CAD build for the part. Positions are in the model's coordinates, mm. Face numbers are marked on the shaded views. Give positions to 0.01 mm unless a question says otherwise; leave off trailing zeros. Loops run counter-clockwise (first coordinate to the right, second up) from the corner with the lowest first, then second, coordinate; pieces in that order, holes last. Notation, with made-up numbers: M 44,-3.5 L 95,-3.5 A11 cw 95,5.5 Z; hole C 56.25,80 d10. An arc over 180 degrees is marked long. One line per question, with ' | ' between items.
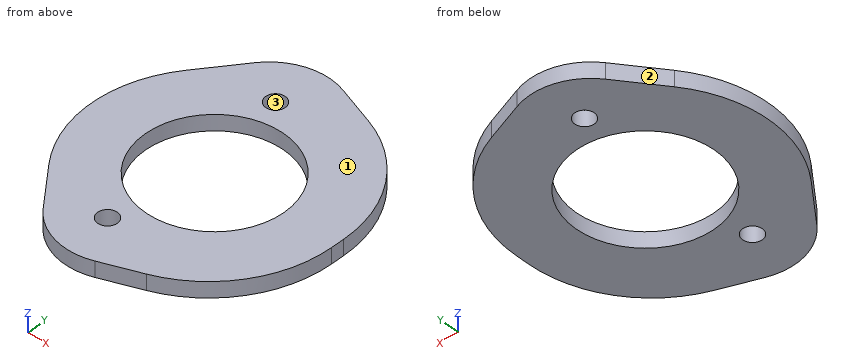
Autodesk Inventor part; units mm, degrees
ref_plane "Work Plane2" through (21.5824, 22.0396, 3.2283) normal (0, 0, 1) x (0.9852, -0.1712, 0)
ref_plane "YZ Plane" through (0, 0, 0) normal (1, 0, 0) x (0, 1, 0)
ref_plane "XZ Plane" through (0, 0, 0) normal (0, 1, 0) x (-1, 0, 0)
ref_plane "Work Plane1" through (0, 0, 0) normal (0, 0, 1) x (1, 0, 0)
sketch "Sketch1" plane through (0, 0, 0) normal (0, 0, 1) x (1, 0, 0)
  line L0 (38.5336, 66.2269) -> (46.4641, 63.2899)
  line L1 (63.0428, 39.4709) -> (63.0428, 36.7291)
  line L2 (46.4641, 12.9101) -> (38.5336, 9.9731)
  line L3 (24.0727, 14.1184) -> (17.5423, 22.5716)
  line L4 (17.5423, 53.6284) -> (24.0727, 62.0816)
  circle A0 centre (37.6428, 38.1) radius 14.2875
  circle A1 centre (32.8676, 57.15) radius 2.0193
  circle A2 centre (32.8676, 19.05) radius 2.0193
  line L5 (37.6428, 38.1) -> (32.8676, 57.15) construction
  line L6 (37.6428, 38.1) -> (32.8676, 19.05) construction
  arc A3 (38.5336, 66.2269) -> (24.0727, 62.0816) centre (34.123, 54.3174) ccw
  arc A4 (24.0727, 14.1184) -> (38.5336, 9.9731) centre (34.123, 21.8826) ccw
  arc A5 (17.5423, 53.6284) -> (17.5423, 22.5716) centre (37.6428, 38.1) ccw
  arc A6 (46.4641, 12.9101) -> (63.0428, 36.7291) centre (37.6428, 36.7291) ccw
  arc A7 (63.0428, 39.4709) -> (46.4641, 63.2899) centre (37.6428, 39.4709) ccw
  line L7 (12.2428, 46.8808) -> (12.2428, 25.1015) construction
  point P0 (29.7797, 69.4689)
  point P1 (63.0428, 57.15)
  point P2 (63.0428, 19.05)
  point P3 (29.7797, 6.7311)
  point P4 (5.5461, 38.1)
  point P5 (63.0428, 38.1)
  dimension "d2" = 12.7
  dimension "d3" = 12.7
  dimension "d5" = 25.4
  dimension "d6" = 38.1
  dimension "d7" = 12.7
  dimension "d8" = 25.4
  dimension "d9" = 25.4
ref_plane "Work Plane2" through (21.5824, 22.0396, 3.2283) normal (0, 0, 1) x (0.9852, -0.1712, 0)
extrude "Extrusion1" add sketch "Sketch1" along normal up to surface (3.2283 mm away)
equation "\"d9\" = d5"
properties part number "Encoder Mount"
Item 1: Saw through at B-B on z = 1.4. State how many separate pieces and enclosed holes the cut face has, and give its area (3 significant figures).
Conclusion:
separate pieces: 1 | enclosed holes: 3 | area: 1,550 mm²
Item 2: Saw through at C-C on x = 32.5. Give the cut face in (y, z), and give its area (3 significant figures).
Conclusion:
outline: M 9.29,0 L 17.06,0 L 17.06,3.23 L 9.29,3.23 Z; M 21.04,0 L 24.77,0 L 24.77,3.23 L 21.04,3.23 Z; M 51.43,0 L 55.16,0 L 55.16,3.23 L 51.43,3.23 Z; M 59.14,0 L 66.91,0 L 66.91,3.23 L 59.14,3.23 Z | area: 74.3 mm²
Item 3: Drill centre lines: line 1 along Y through (x, z) = (33, 2.05); line 2 along X through (y, z) = (40.5, 2.5); line 3 along X through (y, z) = (55.5, 3). Where is each one in solid material? Low to high. Write a range as [from, to].
Conclusion:
line 1: [9.23, 17.04], [21.06, 24.59], [51.61, 55.14], [59.16, 66.97] | line 2: [12.36, 23.56], [51.73, 63.02] | line 3: [18.99, 31.7], [34.03, 57.35]
Item 4: Mould opens along Y. For the marked faces 1, 2 and 3 say: pulls with the +Y half, pulls with the -Y half, needs draft (parallel to the pull), parting line crosses it, or undercut.
Conclusion:
face 1: needs draft | face 2: pulls with the +Y half | face 3: undercut
Item 5: Saw through at A-A on y = 38.1. Give the cut face in (x, z).
Conclusion:
outline: M 12.24,0 L 23.36,0 L 23.36,3.23 L 12.24,3.23 Z; M 51.93,0 L 63.04,0 L 63.04,3.23 L 51.93,3.23 Z
Item 6: Saw through at D-D on x = 40.5. Give the cut face in (y, z), and give its area (3 significant figures).
Conclusion:
outline: M 10.7,0 L 24.1,0 L 24.1,3.23 L 10.7,3.23 Z; M 52.1,0 L 65.5,0 L 65.5,3.23 L 52.1,3.23 Z | area: 86.5 mm²
Item 7: Drop flat-ended pins along their axis: P1, Ø4.5, axis at x = 32.87, y = 57.15, coming from the -Z side; P2, Ø1.5, axis at x = 39, z = 3, coming from the +Y side. Give the stop position or say it passes through.
Conclusion:
P1: z = 0 | P2: y = 66.33
